```python
from build123d import *

# Parameters (mm, degrees)
F1_DEPTH = 6.35
F2_W     = 50.8
F2_H     = 50.8
F3_DEPTH = 3.175


with BuildPart() as f1:
    # F0 (on Top) → F1 (new body)
    with BuildSketch(Plane.XY):
        with BuildLine():
            Line((25.4, 22.225), (25.4, 25.4))
            Line((25.4, 25.4), (22.225, 25.4))
            Line((22.225, 25.4), (22.225, 23.8125))
            ThreePointArc((22.225, 23.8125), (23.3475320151, 23.3475320151), (23.8125, 22.225))
            Line((23.8125, 22.225), (25.4, 22.225))
        make_face()
        with BuildLine():
            Line((22.225, 23.8125), (22.225, 25.4))
            Line((22.225, 25.4), (-22.225, 25.4))
            Line((-22.225, 25.4), (-22.225, 23.8125))
            ThreePointArc((-22.225, 23.8125), (-21.1024679849, 23.3475320151), (-20.6375, 22.225))
            Line((-20.6375, 22.225), (-17.4625, 22.225))
            ThreePointArc((-17.4625, 22.225), (-15.875, 23.8125), (-14.2875, 22.225))
            Line((-14.2875, 22.225), (-11.1125, 22.225))
            ThreePointArc((-11.1125, 22.225), (-9.525, 23.8125), (-7.9375, 22.225))
            Line((-7.9375, 22.225), (-4.7625, 22.225))
            ThreePointArc((-4.7625, 22.225), (-3.175, 23.8125), (-1.5875, 22.225))
            Line((-1.5875, 22.225), (1.5875, 22.225))
            ThreePointArc((1.5875, 22.225), (3.175, 23.8125), (4.7625, 22.225))
            Line((4.7625, 22.225), (7.9375, 22.225))
            ThreePointArc((7.9375, 22.225), (9.525, 23.8125), (11.1125, 22.225))
            Line((11.1125, 22.225), (14.2875, 22.225))
            ThreePointArc((14.2875, 22.225), (15.875, 23.8125), (17.4625, 22.225))
            Line((17.4625, 22.225), (20.6375, 22.225))
            ThreePointArc((20.6375, 22.225), (21.1024679849, 23.3475320151), (22.225, 23.8125))
        make_face()
        with BuildLine():
            Line((25.4, -22.225), (25.4, 22.225))
            Line((25.4, 22.225), (23.8125, 22.225))
            ThreePointArc((23.8125, 22.225), (23.3475320151, 21.1024679849), (22.225, 20.6375))
            Line((22.225, 20.6375), (22.225, 17.4625))
            ThreePointArc((22.225, 17.4625), (23.3475320151, 16.9975320151), (23.8125, 15.875))
            ThreePointArc((23.8125, 15.875), (23.3475320151, 14.7524679849), (22.225, 14.2875))
            Line((22.225, 14.2875), (22.225, 11.1125))
            ThreePointArc((22.225, 11.1125), (23.3475320151, 10.6475320151), (23.8125, 9.525))
            ThreePointArc((23.8125, 9.525), (23.3475320151, 8.4024679849), (22.225, 7.9375))
            Line((22.225, 7.9375), (22.225, 4.7625))
            ThreePointArc((22.225, 4.7625), (23.3475320151, 4.2975320151), (23.8125, 3.175))
            ThreePointArc((23.8125, 3.175), (23.3475320151, 2.0524679849), (22.225, 1.5875))
            Line((22.225, 1.5875), (22.225, -1.5875))
            ThreePointArc((22.225, -1.5875), (23.3475320151, -2.0524679849), (23.8125, -3.175))
            ThreePointArc((23.8125, -3.175), (23.3475320151, -4.2975320151), (22.225, -4.7625))
            Line((22.225, -4.7625), (22.225, -7.9375))
            ThreePointArc((22.225, -7.9375), (23.3475320151, -8.4024679849), (23.8125, -9.525))
            ThreePointArc((23.8125, -9.525), (23.3475320151, -10.6475320151), (22.225, -11.1125))
            Line((22.225, -11.1125), (22.225, -14.2875))
            ThreePointArc((22.225, -14.2875), (23.3475320151, -14.7524679849), (23.8125, -15.875))
            ThreePointArc((23.8125, -15.875), (23.3475320151, -16.9975320151), (22.225, -17.4625))
            Line((22.225, -17.4625), (22.225, -20.6375))
            ThreePointArc((22.225, -20.6375), (23.3475320151, -21.1024679849), (23.8125, -22.225))
            Line((23.8125, -22.225), (25.4, -22.225))
        make_face()
        with BuildLine():
            Line((-22.225, 23.8125), (-22.225, 25.4))
            Line((-22.225, 25.4), (-25.4, 25.4))
            Line((-25.4, 25.4), (-25.4, 22.225))
            Line((-25.4, 22.225), (-23.8125, 22.225))
            ThreePointArc((-23.8125, 22.225), (-23.3475320151, 23.3475320151), (-22.225, 23.8125))
        make_face()
        with BuildLine():
            Line((25.4, -25.4), (25.4, -22.225))
            Line((25.4, -22.225), (23.8125, -22.225))
            ThreePointArc((23.8125, -22.225), (23.3475320151, -23.3475320151), (22.225, -23.8125))
            Line((22.225, -23.8125), (22.225, -25.4))
            Line((22.225, -25.4), (25.4, -25.4))
        make_face()
        with BuildLine():
            Line((-23.8125, 22.225), (-25.4, 22.225))
            Line((-25.4, 22.225), (-25.4, 15.875))
            Line((-25.4, 15.875), (-25.4, 9.525))
            Line((-25.4, 9.525), (-25.4, 3.175))
            Line((-25.4, 3.175), (-25.4, -3.175))
            Line((-25.4, -3.175), (-25.4, -9.525))
            Line((-25.4, -9.525), (-25.4, -15.875))
            Line((-25.4, -15.875), (-25.4, -22.225))
            Line((-25.4, -22.225), (-23.8125, -22.225))
            ThreePointArc((-23.8125, -22.225), (-23.3475320151, -21.1024679849), (-22.225, -20.6375))
            Line((-22.225, -20.6375), (-22.225, -17.4625))
            ThreePointArc((-22.225, -17.4625), (-23.8125, -15.875), (-22.225, -14.2875))
            Line((-22.225, -14.2875), (-22.225, -11.1125))
            ThreePointArc((-22.225, -11.1125), (-23.8125, -9.525), (-22.225, -7.9375))
            Line((-22.225, -7.9375), (-22.225, -4.7625))
            ThreePointArc((-22.225, -4.7625), (-23.8125, -3.175), (-22.225, -1.5875))
            Line((-22.225, -1.5875), (-22.225, 1.5875))
            ThreePointArc((-22.225, 1.5875), (-23.8125, 3.175), (-22.225, 4.7625))
            Line((-22.225, 4.7625), (-22.225, 7.9375))
            ThreePointArc((-22.225, 7.9375), (-23.8125, 9.525), (-22.225, 11.1125))
            Line((-22.225, 11.1125), (-22.225, 14.2875))
            ThreePointArc((-22.225, 14.2875), (-23.8125, 15.875), (-22.225, 17.4625))
            Line((-22.225, 17.4625), (-22.225, 20.6375))
            ThreePointArc((-22.225, 20.6375), (-23.3475320151, 21.1024679849), (-23.8125, 22.225))
        make_face()
        with BuildLine():
            Line((15.875, -25.4), (22.225, -25.4))
            Line((22.225, -25.4), (22.225, -23.8125))
            ThreePointArc((22.225, -23.8125), (21.1024679849, -23.3475320151), (20.6375, -22.225))
            Line((20.6375, -22.225), (17.4625, -22.225))
            ThreePointArc((17.4625, -22.225), (15.875, -23.8125), (14.2875, -22.225))
            Line((14.2875, -22.225), (11.1125, -22.225))
            ThreePointArc((11.1125, -22.225), (9.525, -23.8125), (7.9375, -22.225))
            Line((7.9375, -22.225), (4.7625, -22.225))
            ThreePointArc((4.7625, -22.225), (3.175, -23.8125), (1.5875, -22.225))
            Line((1.5875, -22.225), (-1.5875, -22.225))
            ThreePointArc((-1.5875, -22.225), (-3.175, -23.8125), (-4.7625, -22.225))
            Line((-4.7625, -22.225), (-7.9375, -22.225))
            ThreePointArc((-7.9375, -22.225), (-9.525, -23.8125), (-11.1125, -22.225))
            Line((-11.1125, -22.225), (-14.2875, -22.225))
            ThreePointArc((-14.2875, -22.225), (-15.875, -23.8125), (-17.4625, -22.225))
            Line((-17.4625, -22.225), (-20.6375, -22.225))
            ThreePointArc((-20.6375, -22.225), (-21.1024679849, -23.3475320151), (-22.225, -23.8125))
            Line((-22.225, -23.8125), (-22.225, -25.4))
            Line((-22.225, -25.4), (-15.875, -25.4))
            Line((-15.875, -25.4), (-9.525, -25.4))
            Line((-9.525, -25.4), (-3.175, -25.4))
            Line((-3.175, -25.4), (3.175, -25.4))
            Line((3.175, -25.4), (9.525, -25.4))
            Line((9.525, -25.4), (15.875, -25.4))
        make_face()
        with BuildLine():
            Line((-23.8125, -22.225), (-25.4, -22.225))
            Line((-25.4, -22.225), (-25.4, -25.4))
            Line((-25.4, -25.4), (-22.225, -25.4))
            Line((-22.225, -25.4), (-22.225, -23.8125))
            ThreePointArc((-22.225, -23.8125), (-23.3475320151, -23.3475320151), (-23.8125, -22.225))
        make_face()
        with BuildLine():
            ThreePointArc((22.225, 20.6375), (21.1024679849, 21.1024679849), (20.6375, 22.225))
            Line((20.6375, 22.225), (17.4625, 22.225))
            ThreePointArc((17.4625, 22.225), (15.875, 20.6375), (14.2875, 22.225))
            Line((14.2875, 22.225), (11.1125, 22.225))
            ThreePointArc((11.1125, 22.225), (9.525, 20.6375), (7.9375, 22.225))
            Line((7.9375, 22.225), (4.7625, 22.225))
            ThreePointArc((4.7625, 22.225), (3.175, 20.6375), (1.5875, 22.225))
            Line((1.5875, 22.225), (-1.5875, 22.225))
            ThreePointArc((-1.5875, 22.225), (-3.175, 20.6375), (-4.7625, 22.225))
            Line((-4.7625, 22.225), (-7.9375, 22.225))
            ThreePointArc((-7.9375, 22.225), (-9.525, 20.6375), (-11.1125, 22.225))
            Line((-11.1125, 22.225), (-14.2875, 22.225))
            ThreePointArc((-14.2875, 22.225), (-15.875, 20.6375), (-17.4625, 22.225))
            Line((-17.4625, 22.225), (-20.6375, 22.225))
            ThreePointArc((-20.6375, 22.225), (-21.1024679849, 21.1024679849), (-22.225, 20.6375))
            Line((-22.225, 20.6375), (-22.225, 17.4625))
            ThreePointArc((-22.225, 17.4625), (-21.1024679849, 16.9975320151), (-20.6375, 15.875))
            ThreePointArc((-20.6375, 15.875), (-21.1024679849, 14.7524679849), (-22.225, 14.2875))
            Line((-22.225, 14.2875), (-22.225, 11.1125))
            ThreePointArc((-22.225, 11.1125), (-21.1024679849, 10.6475320151), (-20.6375, 9.525))
            ThreePointArc((-20.6375, 9.525), (-21.1024679849, 8.4024679849), (-22.225, 7.9375))
            Line((-22.225, 7.9375), (-22.225, 4.7625))
            ThreePointArc((-22.225, 4.7625), (-21.1024679849, 4.2975320151), (-20.6375, 3.175))
            ThreePointArc((-20.6375, 3.175), (-21.1024679849, 2.0524679849), (-22.225, 1.5875))
            Line((-22.225, 1.5875), (-22.225, -1.5875))
            ThreePointArc((-22.225, -1.5875), (-21.1024679849, -2.0524679849), (-20.6375, -3.175))
            ThreePointArc((-20.6375, -3.175), (-21.1024679849, -4.2975320151), (-22.225, -4.7625))
            Line((-22.225, -4.7625), (-22.225, -7.9375))
            ThreePointArc((-22.225, -7.9375), (-21.1024679849, -8.4024679849), (-20.6375, -9.525))
            ThreePointArc((-20.6375, -9.525), (-21.1024679849, -10.6475320151), (-22.225, -11.1125))
            Line((-22.225, -11.1125), (-22.225, -14.2875))
            ThreePointArc((-22.225, -14.2875), (-21.1024679849, -14.7524679849), (-20.6375, -15.875))
            ThreePointArc((-20.6375, -15.875), (-21.1024679849, -16.9975320151), (-22.225, -17.4625))
            Line((-22.225, -17.4625), (-22.225, -20.6375))
            ThreePointArc((-22.225, -20.6375), (-21.1024679849, -21.1024679849), (-20.6375, -22.225))
            Line((-20.6375, -22.225), (-17.4625, -22.225))
            ThreePointArc((-17.4625, -22.225), (-15.875, -20.6375), (-14.2875, -22.225))
            Line((-14.2875, -22.225), (-11.1125, -22.225))
            ThreePointArc((-11.1125, -22.225), (-9.525, -20.6375), (-7.9375, -22.225))
            Line((-7.9375, -22.225), (-4.7625, -22.225))
            ThreePointArc((-4.7625, -22.225), (-3.175, -20.6375), (-1.5875, -22.225))
            Line((-1.5875, -22.225), (1.5875, -22.225))
            ThreePointArc((1.5875, -22.225), (3.175, -20.6375), (4.7625, -22.225))
            Line((4.7625, -22.225), (7.9375, -22.225))
            ThreePointArc((7.9375, -22.225), (9.525, -20.6375), (11.1125, -22.225))
            Line((11.1125, -22.225), (14.2875, -22.225))
            ThreePointArc((14.2875, -22.225), (15.875, -20.6375), (17.4625, -22.225))
            Line((17.4625, -22.225), (20.6375, -22.225))
            ThreePointArc((20.6375, -22.225), (21.1024679849, -21.1024679849), (22.225, -20.6375))
            Line((22.225, -20.6375), (22.225, -17.4625))
            ThreePointArc((22.225, -17.4625), (20.6375, -15.875), (22.225, -14.2875))
            Line((22.225, -14.2875), (22.225, -11.1125))
            ThreePointArc((22.225, -11.1125), (20.6375, -9.525), (22.225, -7.9375))
            Line((22.225, -7.9375), (22.225, -4.7625))
            ThreePointArc((22.225, -4.7625), (20.6375, -3.175), (22.225, -1.5875))
            Line((22.225, -1.5875), (22.225, 1.5875))
            ThreePointArc((22.225, 1.5875), (20.6375, 3.175), (22.225, 4.7625))
            Line((22.225, 4.7625), (22.225, 7.9375))
            ThreePointArc((22.225, 7.9375), (20.6375, 9.525), (22.225, 11.1125))
            Line((22.225, 11.1125), (22.225, 14.2875))
            ThreePointArc((22.225, 14.2875), (20.6375, 15.875), (22.225, 17.4625))
            Line((22.225, 17.4625), (22.225, 20.6375))
        make_face()
    extrude(amount=F1_DEPTH)

    # F2 (on face) → F3 (join)
    with BuildSketch(Plane(origin=(0, 0, 0), x_dir=(1, 0, 0), z_dir=(0, 0, -1))):
        Rectangle(F2_W, F2_H)
    extrude(amount=F3_DEPTH)


solid = f1.part
```
Source: CAD feature listing. Evaluate the final solid. Frame: model axes, mm. A direction names the side the tool comes from. Round coordinates to 2 decimals unless told otherwise and drop trailing zeros. Loops run counter-clockwise (first coordinate to the right, second up) from the corner with the lowest first, then second, coordinate; pieces in that order, holes last.
(1) Contact query for flat-ended pins moving along their axis: pin 1 Ø1 at (x, y) = (22, 16) entering from +Z; pin 2 Ø2.5 at (x, y) = (10.5, 22) entering from +Z. Output: stop coordinate, or through.
From the geometry:
pin 1: stops at z = 0
pin 2: stops at z = 6.35
(2) Section query B-B (y = 10.5). Output: boundary loops of the cut face in (x, z) (3 decimals), and give its area (3 significant figures).
From the geometry:
outline: (-25.4, -3.175) - (25.4, -3.175) - (25.4, 6.35) - (23.478, 6.35) - (23.478, 0) - (20.972, 0) - (20.972, 6.35) - (-20.972, 6.35) - (-20.972, 0) - (-23.478, 0) - (-23.478, 6.35) - (-25.4, 6.35) - close
area: 452 mm2
(3) Pull-direction query (X, two-part tool) for faces 3 (the flat face through (0, 0, -3.175)), 4 (the flat face through (22, 10, 0)); classes: +X half, -X half, draft (parallel to the pull), parting line (faces both ways), or undercut.
From the geometry:
face 3: draft
face 4: undercut
(4) Access query for faces 1 (the flat face through (0, -25.4, 2)), 2 (the cylindrical face through (9.73, -20.65, 3.13)). Directions: +Z, -Z, +X, -X, +Y, -Y. A direction counts if a zero-diameter tool reaches every point of the face in a straight line with its end or side. Return the directions, or none.
From the geometry:
face 1: +Z, -Z, +X, -X, -Y
face 2: +Z
(5) Material intervals for probe 1 along X at (y, z) = (-16, 1); probe 2 along Y at (x, z) = (-17, 3), sorted ascending.
From the geometry:
probe 1: x = -25.4 to -23.81, -20.64 to 20.64, 23.81 to 25.4
probe 2: y = -25.4 to -23.35, -21.1 to 21.1, 23.35 to 25.4
(6) Section query A-A (z = 2.25). Give the number of separate pieces and of enclosed holes in the cut face, and give its area (3 significant figures).
From the geometry:
separate pieces: 1
enclosed holes: 28
area: 2,360 mm2
